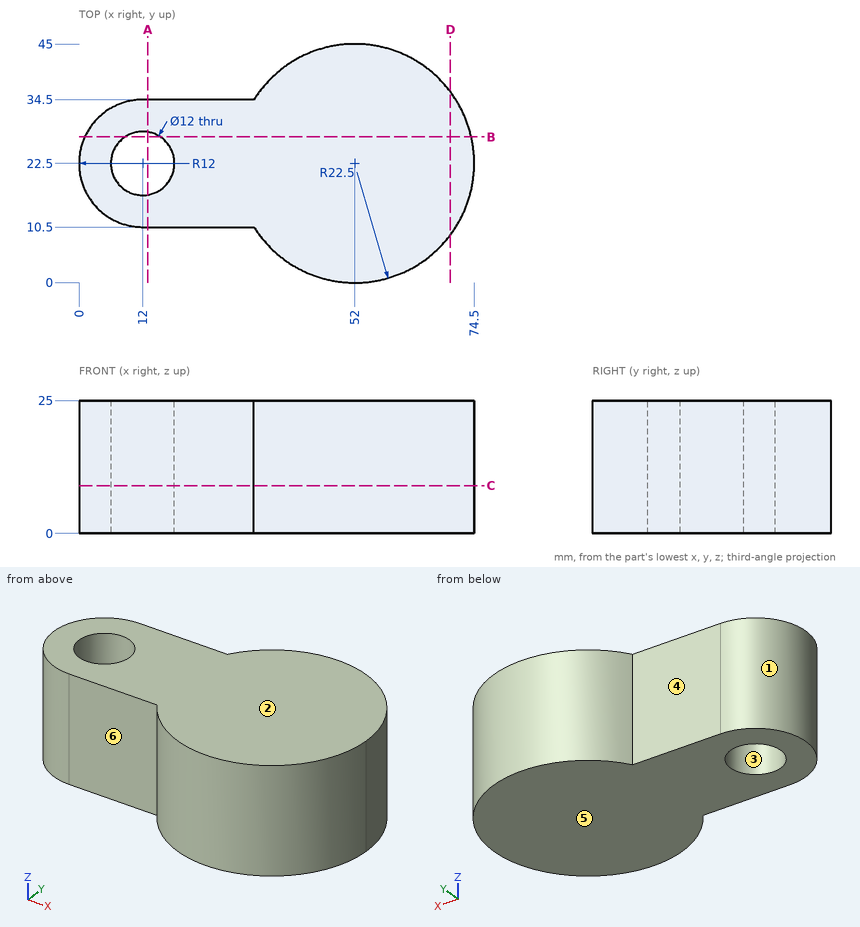
Here's the drawing with two shaded views (mm, measured from the low corner). I have some questions. A direction names the side the tool comes from. Give positions to 0.01 mm unless a question says otherwise; leave off trailing zeros. Write each loop counter-clockwise with the first axis right and the second up, starting at its lowest first coordinate (ties: lowest second). Pieces come first, ordered by that corner, then holes. Notation, with made-up numbers: (42, 75.25) -> (86, 75.25) arc R18 cw to (86, 90.25) -> close; hole circle Ø9 at (1, 14). An arc over 180 degrees is marked (long way). One line per item, written item: value.
Q1. Which directions (+Z, -Z, +X, -X, +Y, -Y) give clear straight access to the entire face, cutting with the end or side of a thin tool? Please do the marked faces 4, 5 and 6.
Results found:
face 4: +Z, -Z, -X, +Y
face 5: -Z, +X, -X, +Y, -Y
face 6: +Z, -Z, -X, -Y
Q2. Please list where these lines run through material, in increasing order: line 1 (Y direction, x = 12, z = 12.75); line 2 (Y direction, x = 27, z = 13); line 3 (X direction, y = 17.5, z = 18.5). Write a range as [from, to].
Results found:
line 1: y = [10.5, 16.5], [28.5, 34.5]
line 2: y = [10.5, 34.5]
line 3: x = [1.09, 8.68], [15.32, 73.94]
Q3. Imagine slicing it at A-A on x = 13. Please give me the cut outline in (y, z), and give its area (3 significant figures).
Results found:
outline: (10.5, 0) -> (16.58, 0) -> (16.58, 25) -> (10.5, 25) -> close; (28.42, 0) -> (34.5, 0) -> (34.5, 25) -> (28.42, 25) -> close
area: 304 mm^2
Q4. Imagine slicing it at D-D on x = 70. Please give me the cut outline in (y, z).
Results found:
outline: (9, 0) -> (36, 0) -> (36, 25) -> (9, 25) -> close
Q5. Imagine slicing it at C-C on z = 9. Please give me the cut outline in (x, y), and give its area (3 significant figures).
Results found:
outline: (12, 10.5) -> (32.97, 10.5) arc R22.5 ccw to (74.5, 22.5) arc R22.5 ccw to (32.97, 34.5) -> (12, 34.5) arc R12 ccw to start; hole circle Ø12 at (12, 22.5)
area: 2,150 mm^2
Q6. We'd pull the mould along X, two halves only. Please class the marked faces 1, 2 and 3: +X half, -X half, draft (parallel to the pull), parting line (faces both ways), or undercut.
Results found:
face 1: -X half
face 2: draft
face 3: undercut
Q7. For P1, Ø4, axis at y = 29, z = 15.5, coming from the -X side; P2, Ø4, axis at x = 62.5, z = 15.5, coming from the +Y side; P3, Ø5, axis at x = 65, z = 5, coming from the +Y side; P4, Ø3, axis at x = 30, y = 29, coming from the -Z side, each with a flat end and sliding along its axis, tell me the tip position at first contact or that it passes through.
Results found:
P1: stops at x = 0.88
P2: stops at y = 43.33
P3: stops at y = 42.4
P4: stops at z = 0
Q8. Imagine slicing it at B-B on y = 27.5. Please give me the cut outline in (x, z), and give its area (3 significant figures).
Results found:
outline: (1.09, 0) -> (8.68, 0) -> (8.68, 25) -> (1.09, 25) -> close; (15.32, 0) -> (73.94, 0) -> (73.94, 25) -> (15.32, 25) -> close
area: 1,660 mm^2
